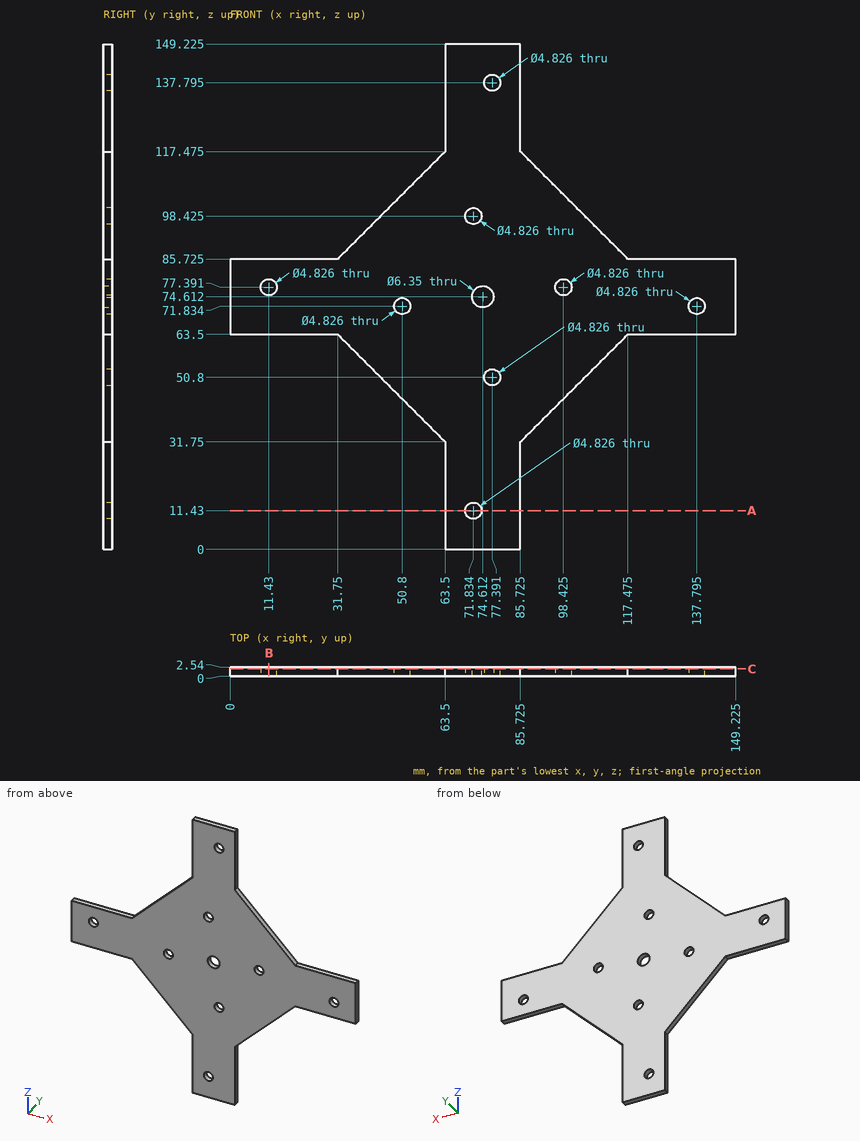
Could you check a few things on this drawing? It's one solid part, dimensions in mm from its lowest x, y, z. Coordinates: 2 decimals unless noted, no trailing zeros. Order: outer loops, then holes, each group sorted by start corner. A loop starts at its lowest first (then second) coordinate and runs counter-clockwise, first axis right, second up. Notation, with made-up numbers: M 54.5,71.5 L 87.5,71.5 A27 cw 87.5,87.5 Z; hole C 3.5,33 d7. An arc over 180 degrees is marked long. Answer as a JSON object with one key per item and string values. Group by question number.
(1) Suppose I cut it at C-C, the plane y = 2.1. State how many separate pieces and enclosed holes the cut face has, then the cut area to 3 significant figures.
(2) Suppose I cut it at B-B, the plane x = 11.43. Please give me the cut outline in (y, z) (1 decimal).
(3) I need wall thicknesses on probe 1 along X at (y, z) = (2.35, 11) (1 decimal); probe 2 along Z at (x, y) = (138, 2.05) (1 decimal); probe 3 along Z at (x, y) = (30.5, 2.45) (1 decimal). Which ranges of each line are inside material? Lowest first, please.
(4) For pin 1 (7.5 mm diameter, centred on x = 50.8, z = 71.83, fed in from +Y); pin 2 (1.3 mm diameter, centred on x = 141, y = 1, fed in from -Z); pin 3 (0.8 mm diameter, centred on x = 132, y = 1.5, fed in from +Z) (1 decimal); pin 4 (4 mm diameter, centred on x = 98.42, z = 77.39, fed in from -Y), each with a flat end and sliding along its axis, tell me the tip position at first contact or that it passes through.
(5) Suppose I cut it at A-A, the plane z = 11.43. Please give me the cut outline in (x, y) (1 decimal).
Values found:
{
 "1": {"separate pieces": "1", "enclosed holes": "9", "area": "7,980 mm^2"},
 "2": {"outline": "M 0,63.5 L 2.5,63.5 L 2.5,75 L 0,75 Z; M 0,79.8 L 2.5,79.8 L 2.5,85.7 L 0,85.7 Z"},
 "3": {"probe 1": "x = 63.5 to 69.5, 74.2 to 85.7", "probe 2": "z = 63.5 to 69.4, 74.2 to 85.7", "probe 3": "z = 63.5 to 85.7"},
 "4": {"pin 1": "stops at y = 2.54", "pin 2": "stops at z = 63.5", "pin 3": "stops at z = 85.7", "pin 4": "passes through"},
 "5": {"outline": "M 63.5,0 L 69.4,0 L 69.4,2.5 L 63.5,2.5 Z; M 74.2,0 L 85.7,0 L 85.7,2.5 L 74.2,2.5 Z"}
}
